from build123d import *

# Parameters (mm, degrees)
ESQUISSE1_W             = 100
ESQUISSE1_H             = 80
BOSS_EXTRU_1_DEPTH      = 20
COQUE1_T                = -1.5
CONG_1_R                = 5
ESQUISSE3_W             = 90
ESQUISSE3_H             = 20
ENL_V_MAT_EXTRU_2_DEPTH = 20
CONG_5_R                = 20
CONG_6_R                = 0.5


with BuildPart() as part:
    # Esquisse1 → Boss.-Extru.1 (new body)
    with BuildSketch(Plane.XY):
        Rectangle(ESQUISSE1_W, ESQUISSE1_H)
    extrude(amount=BOSS_EXTRU_1_DEPTH)

    # Coque1
    coque1_openings = [part.faces().sort_by_distance(p)[0] for p in [
        (0, 0, 0),
    ]]
    offset(amount=COQUE1_T, openings=coque1_openings, kind=Kind.INTERSECTION)

    # Congé1
    cong_1_edges = [part.edges().sort_by_distance(p)[0] for p in [
        (50, -40, 10),
        (-50, -40, 10),
        (-50, 40, 10),
        (50, 40, 10),
    ]]
    fillet(cong_1_edges, radius=CONG_1_R)

    # Esquisse3 → Enlèv. mat.-Extru.2 (cut)
    with BuildSketch(Plane(origin=(0, 40, 0), x_dir=(1, 0, 0), z_dir=(0, 1, 0))):
        with Locations((0, -10)):
            Rectangle(ESQUISSE3_W, ESQUISSE3_H)
    extrude(amount=-ENL_V_MAT_EXTRU_2_DEPTH, mode=Mode.SUBTRACT)

    # Congé5
    # the kernel refuses this fillet: 20 mm, written as the material it takes off along each edge
    with BuildSketch(Plane(origin=(-45, 20, 18.5), x_dir=(0, 0, 1), z_dir=(1, 0, 0))) as cong_5_piece_1:
        with BuildLine():
            CenterArc((20, 7.599342077), CONG_5_R, 180, 22.331645009)
            Line((0, 7.599342077), (0, 0))
            Line((0, 0), (1.5, 0))
        make_face()
    extrude(amount=90, mode=Mode.SUBTRACT)

    # Congé6
    cong_6_edges = [part.edges().sort_by_distance(p)[0] for p in [
        (45, 25.450328962, 18.5),
        (0, 20, 20),
        (-45, 25.450328962, 18.5),
    ]]
    fillet(cong_6_edges, radius=CONG_6_R)


solid = part.part
Geometry check sheet. Reference: the model listing, model coordinates, mm. A direction names the side the tool comes from. Coordinates: 2 decimals unless noted, no trailing zeros. Loops run counter-clockwise (first coordinate to the right, second up) from the corner with the lowest first, then second, coordinate; pieces in that order, holes last. Notation, with made-up numbers: (38, 44.5) - (63, 44.5) arc R15 ccw to (63, 59.5) - close; hole circle Ø9 at (35, -10). An arc over 180 degrees is marked (long way). Use one line per item in the form item = value. Start each with the question number.
Item 1: Section check A-A, the plane y = 31.5. Enter the section's corners in (x, z).
Item 2: Thickness scan on probe 1 along X at (y, z) = (-33.5, 6.75); probe 2 along Z at (x, y) = (-23, 7); probe 3 along Y at (x, z) = (-9.5, 5.25). Record the ranges inside material, lowest first.
Item 3: Tool access check on faces 4 (the face through (-50, 0, 10)), 5 (the face through (48.5, -1, 9)), 6 (the face through (-0.637, 14.634, 18.625)). Record the directions out of +Z, -Z, +X, -X, +Y, -Y that give a thin tool (end or side, any length) a straight path to the whole face; none if there is none.
Item 4: Mould release check, pull along Y, two halves, no side actions. Record for faces 1 (the face through (-45, 39, 13)), 2 (the face through (-49, -38, 10)), 3 (the face through (-48.5, -1, 9)): +Y half, -Y half, draft (parallel to the pull), parting line (faces both ways), or undercut.
Item 5: Section check C-C, the plane y = -21.5. Enter the section's corners in (x, z).
Item 6: Gauge pin test, flat ends, axial feed: pin 1 (6 mm diameter, centred on x = 37, y = 21, fed in from -Z); pin 2 (4 mm diameter, centred on x = 47.5, z = 8.5, fed in from -Y); pin 3 (1.5 mm diameter, centred on x = -2, y = 15.5, fed in from -Z); pin 4 (12 mm diameter, centred on x = 30.5, z = 12, fed in from +Y). Record the tip position at first contact, or that the pin passes through.
Item 7: Section check D-D, the plane x = 19.5. Enter the section's corners in (y, z), and give its area (3 significant figures).
Item 8: Section check B-B, the plane z = 13.5. Enter the section's corners in (x, y).
Computed:
q1.outline = (-50, 0) - (-48.5, 0) - (-48.5, 18.5) - (-45.5, 18.5) arc R0.5 ccw to (-45, 19) - (-45, 20) - (-50, 20) - close; (45, 19) arc R0.5 ccw to (45.5, 18.5) - (48.5, 18.5) - (48.5, 0) - (50, 0) - (50, 20) - (45, 20) - close
q2.probe_1 = -50 to -48.5, 48.5 to 50
q2.probe_2 = 18.5 to 20
q2.probe_3 = -40 to -38.5
q3.face_4 = +Z, -Z, -X, +Y, -Y
q3.face_5 = -Z
q3.face_6 = -Z, +Y
q4.face_1 = draft
q4.face_2 = -Y half
q4.face_3 = undercut
q5.outline = (-50, 0) - (-48.5, 0) - (-48.5, 18.5) - (48.5, 18.5) - (48.5, 0) - (50, 0) - (50, 20) - (-50, 20) - close
q6.pin_1 = through
q6.pin_2 = -39.97
q6.pin_3 = 18.64
q6.pin_4 = -38.5
q7.outline = (-40, 0) - (-38.5, 0) - (-38.5, 18.5) - (12.4, 18.5) arc R20 ccw to (16.9, 19.01) arc R0.5 ccw to (16.79, 20) - (-40, 20) - close
q7.area = 113 mm2
q8.outline = (-50, -35) arc R5 ccw to (-45, -40) - (45, -40) arc R5 ccw to (50, -35) - (50, 35) arc R5 ccw to (45, 40) - (45, 38.5) - (48.5, 38.5) - (48.5, -38.5) - (-48.5, -38.5) - (-48.5, 38.5) - (-45, 38.5) - (-45, 40) arc R5 ccw to (-50, 35) - close
